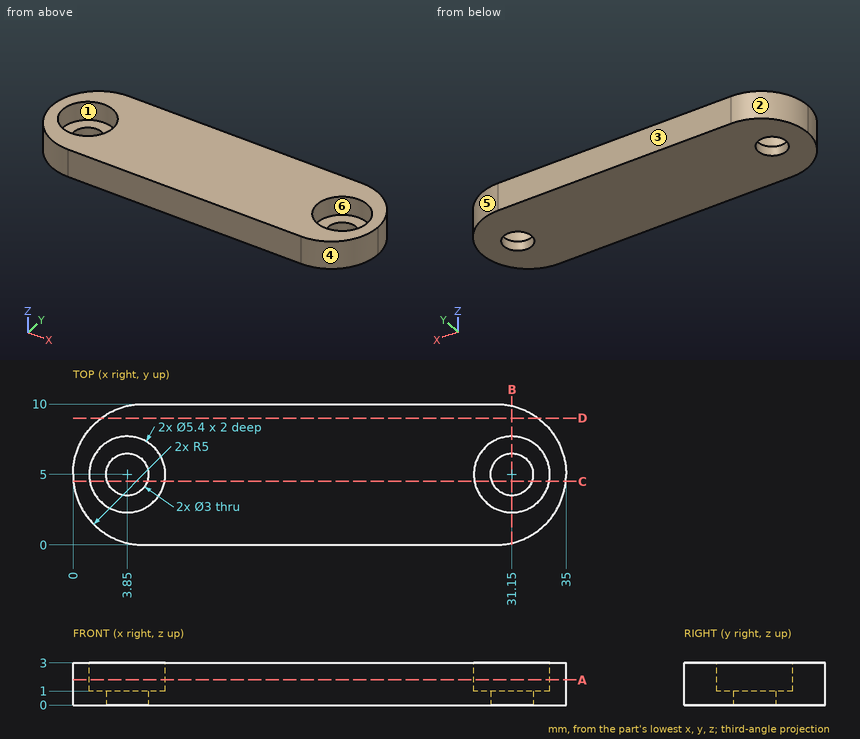
Geometry check sheet. Reference: drawing and pictorial views, mm from the part's lowest x, y, z. A direction names the side the tool comes from. Give positions to 0.01 mm unless a question says otherwise; leave off trailing zeros. Order: outer loops, then holes, each group sorted by start corner. A loop starts at its lowest first (then second) coordinate and runs counter-clockwise, first axis right, second up. Notation, with made-up numbers: (-5.75, 40.25) - (28.25, 40.25) arc R33 ccw to (28.25, 68.25) - close; hole circle Ø4 at (-18.5, 82). An arc over 180 degrees is marked (long way). Use one line per item in the form item = value.
1) Sectioned sample at D-D (y = 9). Record the boundary of the cut face in (x, z), and give its area (3 significant figures).
Working result:
outline = (2, 0) - (33, 0) - (33, 3) - (2, 3) - close
area = 93.0 mm^2
2) Draft check along X on the marked faces 1, 2, 3 and 4. Enter one of: released by +X, released by -X, zero draft, split by the parting line, or undercut.
Working result:
face_1 = undercut
face_2 = released by -X
face_3 = zero draft
face_4 = released by +X
3) Material ranges on probe 1 along X at (y, z) = (4.75, 1.8); probe 2 along X at (y, z) = (4, 2.8); probe 3 along Y at (x, z) = (33.5, 1.4), recorded low to high. Write a range as from..to.
Working result:
probe_1 = 0.01..1.16, 6.54..28.46, 33.84..34.99
probe_2 = 0.1..1.34, 6.36..28.64, 33.66..34.9
probe_3 = 1.43..3.67, 6.33..8.57
4) Sectioned sample at C-C (y = 4.5). Record the boundary of the cut face in (x, z), and give its area (3 significant figures).
Working result:
outline = (0.03, 0) - (2.44, 0) - (2.44, 1) - (1.2, 1) - (1.2, 3) - (0.03, 3) - close; (5.26, 0) - (29.74, 0) - (29.74, 1) - (28.5, 1) - (28.5, 3) - (6.5, 3) - (6.5, 1) - (5.26, 1) - close; (32.56, 0) - (34.97, 0) - (34.97, 3) - (33.8, 3) - (33.8, 1) - (32.56, 1) - close
area = 78.0 mm^2
5) Sectioned sample at A-A (z = 1.8). Count the separate pieces of the cut face and the enclosed holes in it, and give its area (3 significant figures).
Working result:
separate_pieces = 1
enclosed_holes = 2
area = 283 mm^2
6) Sectioned sample at B-B (x = 31.15). Record the boundary of the cut face in (y, z), and give its area (3 significant figures).
Working result:
outline = (0.13, 0) - (3.5, 0) - (3.5, 1) - (2.3, 1) - (2.3, 3) - (0.13, 3) - close; (6.5, 0) - (9.87, 0) - (9.87, 3) - (7.7, 3) - (7.7, 1) - (6.5, 1) - close
area = 15.4 mm^2
7) Access from +Z, -Z, +X, -X, +Y, -Y to the whole of each face (thin tool, end or side, straight path). Record for the marked faces 5 and 6.
Working result:
face_5 = +Z, -Z, +X, +Y
face_6 = +Z
8) Depth check by flat-ended pin: pin 1 Ø1.8 at (x, y) = (3.85, 5) entering from +Z; pin 2 Ø1.5 at (y, z) = (1, 2.5) entering from +X; pin 3 Ø6 at (x, y) = (9.5, 6) entering from -Z; pin 4 Ø4.5 at (x, y) = (31.15, 5) entering from +Z. Enter the tip coordinate at first touch or a pass-through.
Working result:
pin_1 = through
pin_2 = 33.8
pin_3 = 0
pin_4 = 1
